Verification items for this drawing (mm, ordinates from the low corner). A direction names the side the tool comes from. Round coordinates to 2 decimals unless told otherwise and drop trailing zeros. Order: outer loops, then holes, each group sorted by start corner. A loop starts at its lowest first (then second) coordinate and runs counter-clockwise, first axis right, second up. Notation, with made-up numbers: (-8, 13) - (20, 13) arc R34 ccw to (20, 45) - close; hole circle Ø10 at (33.5, 42.25). An arc over 180 degrees is marked (long way). Use a Markdown table: item, result. Add a question column.
(1) Thickness scan on line 1 along X through (y, z) = (20.5, 5); line 2 along Z through (x, y) = (64, 76); line 3 along X through (y, z) = (71, 21). Record the ranges inside material, lowest first. Write a range as [from, to].
(2) Section check D-D on y = 105. Record the boundary of the cut face in (x, z).
(3) Gauge pin test, flat ends, axial feed: P1, Ø2, axis at y = 110, z = 11, coming from the -X side; P2, Ø6, axis at y = 46, z = 8.5, coming from the -X side; P3, Ø11.5, axis at y = 76.2, z = 15.875, coming from the -X side; P4, Ø8, axis at y = 48.5, z = 10.5, coming from the +X side. Record the tip position at first contact, or that the pin passes through.
(4) Section check A-A on y = 76.2. Record the boundary of the cut face in (x, z) (3 decimals).
(5) Access from +Z, -Z, +X, -X, +Y, -Y to the whole of each face (thin tool, end or side, straight path). Record for the marked faces 1, 2, 3 and 4.
(6) Section check C-C on z = 4. Record the boundary of the cut face in (x, y) (3 decimals), then the cut area to 3 significant figures.
(7) Section check B-B on x = 21. Record the boundary of the cut face in (y, z) (3 decimals).
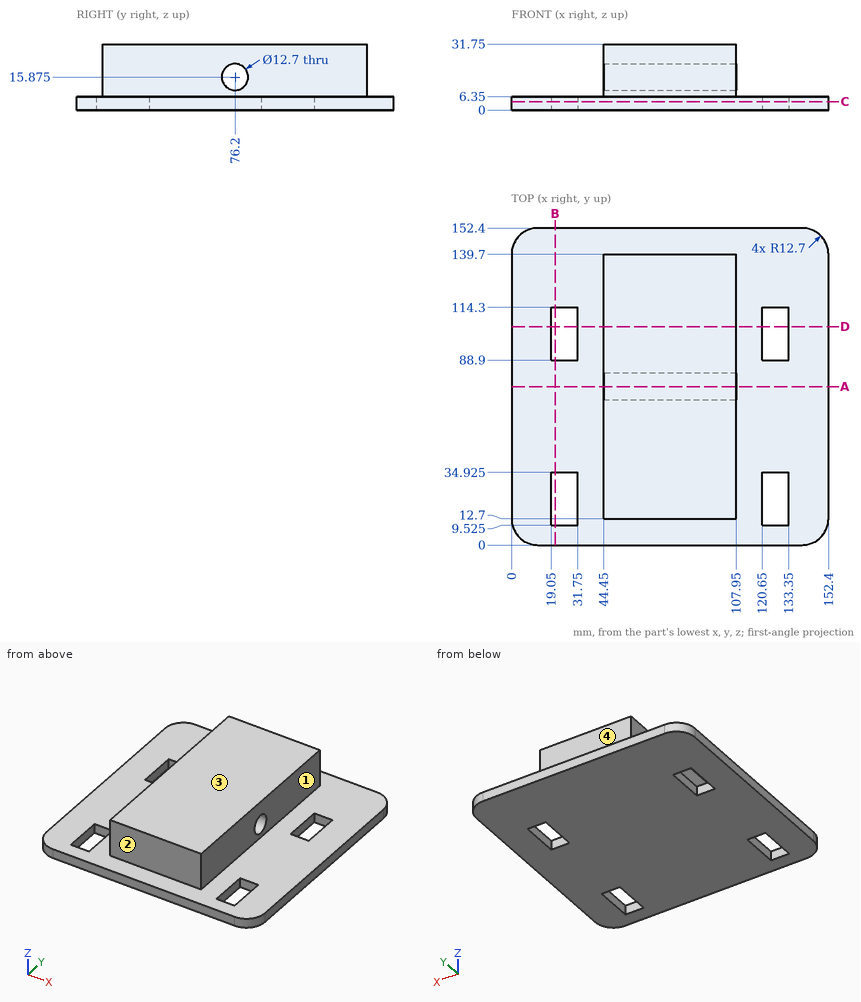
Check sheet entries:
| question | item | result |
|---|---|---|
| 1 | line 1 | x = [0, 19.05], [31.75, 120.65], [133.35, 152.4] |
| 1 | line 2 | z = [0, 9.53], [22.22, 31.75] |
| 1 | line 3 | x = [44.45, 107.95] |
| 2 | outline | (0, 0) - (19.05, 0) - (19.05, 6.35) - (0, 6.35) - close; (31.75, 0) - (120.65, 0) - (120.65, 6.35) - (107.95, 6.35) - (107.95, 31.75) - (44.45, 31.75) - (44.45, 6.35) - (31.75, 6.35) - close; (133.35, 0) - (152.4, 0) - (152.4, 6.35) - (133.35, 6.35) - close |
| 3 | P1 | stops at x = 44.45 |
| 3 | P2 | stops at x = 0 |
| 3 | P3 | passes through |
| 3 | P4 | stops at x = 107.95 |
| 4 | outline | (0, 0) - (152.4, 0) - (152.4, 6.35) - (107.95, 6.35) - (107.95, 9.525) - (44.45, 9.525) - (44.45, 6.35) - (0, 6.35) - close; (44.45, 22.225) - (107.95, 22.225) - (107.95, 31.75) - (44.45, 31.75) - close |
| 5 | face 1 | +Z, +X, +Y, -Y |
| 5 | face 2 | +Z, +X, -X, -Y |
| 5 | face 3 | +Z, +X, -X, +Y, -Y |
| 5 | face 4 | +Z, +X, -X, +Y |
| 6 | outline | (0, 12.7) arc R12.7 ccw to (12.7, 0) - (139.7, 0) arc R12.7 ccw to (152.4, 12.7) - (152.4, 139.7) arc R12.7 ccw to (139.7, 152.4) - (12.7, 152.4) arc R12.7 ccw to (0, 139.7) - close; hole (19.05, 9.525) - (31.75, 9.525) - (31.75, 34.925) - (19.05, 34.925) - close; hole (19.05, 88.9) - (31.75, 88.9) - (31.75, 114.3) - (19.05, 114.3) - close; hole (120.65, 9.525) - (133.35, 9.525) - (133.35, 34.925) - (120.65, 34.925) - close; hole (120.65, 88.9) - (133.35, 88.9) - (133.35, 114.3) - (120.65, 114.3) - close |
| 6 | area | 21,800 mm2 |
| 7 | outline | (0, 0) - (9.525, 0) - (9.525, 6.35) - (0, 6.35) - close; (34.925, 0) - (88.9, 0) - (88.9, 6.35) - (34.925, 6.35) - close; (114.3, 0) - (152.4, 0) - (152.4, 6.35) - (114.3, 6.35) - close |
